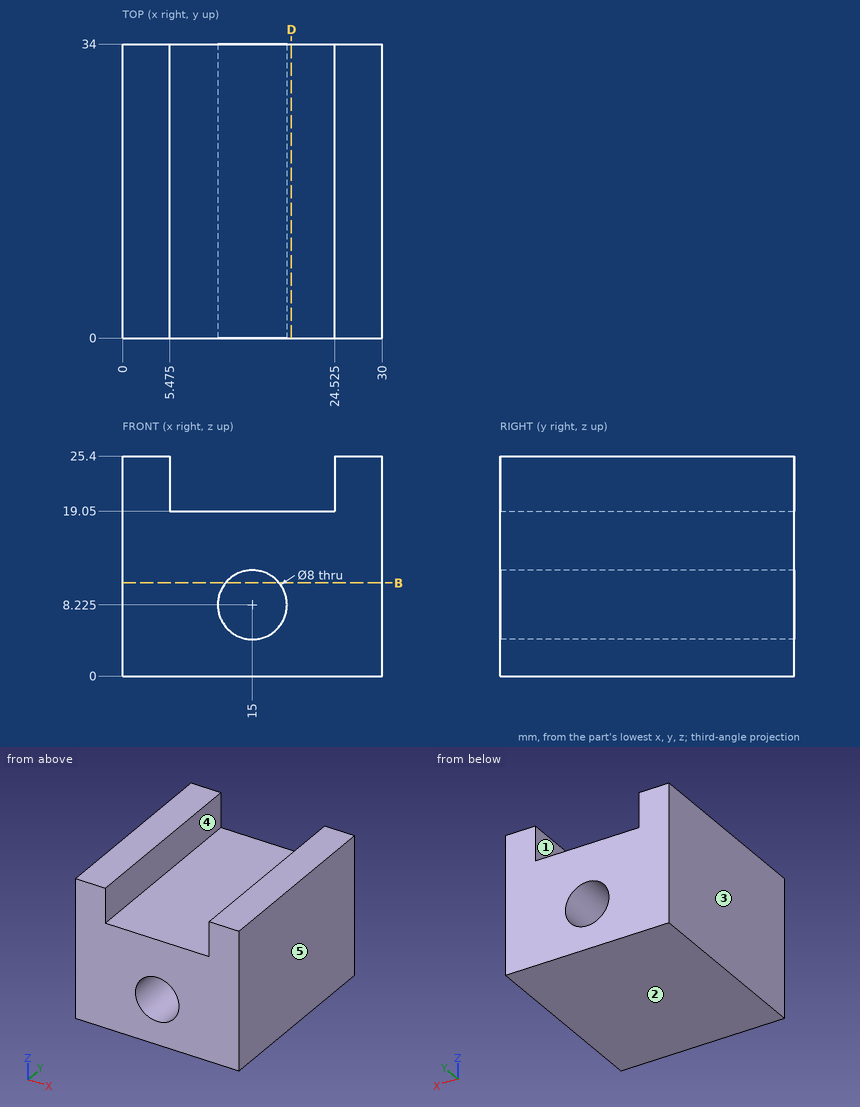
For this review, use the dimensioned drawing (mm, ordinates from the lowest corner) and the shaded views. A direction names the side the tool comes from. Round coordinates to 2 decimals unless told otherwise and drop trailing zeros. Order: outer loops, then holes, each group sorted by start corner. A loop starts at its lowest first (then second) coordinate and runs counter-clockwise, first axis right, second up. Notation, with made-up numbers: (3.25, 58.25) -> (13.25, 58.25) arc R15 ccw to (13.25, 84.25) -> close; hole circle Ø7 at (-11.5, 8.25). An arc over 180 degrees is marked (long way). Put each result on its own line as item: value.
Q1. Add section B-B on z = 10.75. Write out the cut boundary in (x, y).
Check result:
outline: (0, 0) -> (11.9, 0) -> (11.9, 34) -> (0, 34) -> close; (18.1, 0) -> (30, 0) -> (30, 34) -> (18.1, 34) -> close
Q2. For probe 1 along X at (y, z) = (5, 8.25); probe 2 along X at (y, z) = (6, 22.75) (1 decimal); probe 3 along Z at (x, y) = (21, 28), list the stretches that pass through material, from the lowest coordinate up. Write a range as [from, to].
Check result:
probe 1: [0, 11], [19, 30]
probe 2: [0, 5.5], [24.5, 30]
probe 3: [0, 19.05]
Q3. Mouldability with a two-part tool opening along X and no side actions: class the marked faces 3, 4 and 5 as pulls with the +X half, pulls with the -X half, needs draft (parallel to the pull), parting line crosses it, or undercut.
Check result:
face 3: pulls with the -X half
face 4: undercut
face 5: pulls with the +X half
Q4. Machinability: for the marked faces 1 and 2, which of the approach directions +Z, -Z, +X, -X, +Y, -Y give a long, thin tool a straight path to every point of the face, cutting with its end or side? Answer none if there is none.
Check result:
face 1: +Z, +Y, -Y
face 2: -Z, +X, -X, +Y, -Y
Q5. Insertion check: pin 1 Ø13 at (x, z) = (15, 8.22) entering from +Y; pin 2 Ø2 at (x, y) = (21, 5.5) entering from +Z. Each pin has a flat end and moves straight along its axis. Give the tip position at first contact, or say it passes through.
Check result:
pin 1: y = 34
pin 2: z = 19.05
Q6. Add section D-D on x = 19.5. Write out the cut boundary in (y, z).
Check result:
outline: (0, 0) -> (34, 0) -> (34, 19.05) -> (0, 19.05) -> close
